from build123d import *

# Parameters (mm, degrees)
F0_R     = 25.4
F1_DEPTH = 12.7


with BuildPart() as f1:
    # F0 (on Front) → F1 (new body)
    with BuildSketch(Plane.XZ):
        with BuildLine():
            Line((31.8990597447, -65.5396825397), (36.8832878298, -2.9365079365))
            ThreePointArc((36.8832878298, -2.9365079365), (0, 37), (-36.8832878298, -2.9365079365))
            Line((-36.8832878298, -2.9365079365), (-31.8990597447, -65.5396825397))
            ThreePointArc((-31.8990597447, -65.5396825397), (0, -95), (31.8990597447, -65.5396825397))
        make_face()
        with BuildLine():
            Line((-17, -64.5), (-17, -61.5))
            ThreePointArc((-17, -61.5), (0, -44.5), (17, -61.5))
            Line((17, -61.5), (17, -64.5))
            ThreePointArc((17, -64.5), (0, -81.5), (-17, -64.5))
        make_face(mode=Mode.SUBTRACT)
        Circle(F0_R, mode=Mode.SUBTRACT)
    extrude(amount=F1_DEPTH)


solid = f1.part
Model file for the job. Use its own axes, mm. A direction names the side the tool comes from. Give positions to 0.01 mm unless a question says otherwise; leave off trailing zeros. Loops run counter-clockwise (first coordinate to the right, second up) from the corner with the lowest first, then second, coordinate; pieces in that order, holes last. Notation, with made-up numbers: (-12, 51.25) -> (25, 51.25) arc R12 ccw to (25, 66.25) -> close; hole circle Ø3 at (72, 46.5). An arc over 180 degrees is marked (long way). Use a Markdown table: item, result. Add a question column.
(1) Drop flat-ended pins along their axis: pin 1 Ø3 at (x, y) = (-5.5, -1.5) entering from +Z; pin 2 Ø2 at (y, z) = (-6, -24.5) entering from -X; pin 3 Ø2 at (x, y) = (9.5, -6.5) entering from +Z. Give the stop position or say it passes through.
(2) Slice it at B-B on z = -78. List the corners of the cut face in (x, y).
(3) Slice it at A-A on x = 0. List the corners of the cut face in (y, z).
(4) Mould opens along X. For faces 3 (the cylindrical face through (-5.506, -6.261, -24.796)), 4 (the flat face through (-1, 0, -28)), 5 (the cylindrical face through (0.374, -6.261, -81.496)), 6 (the cylindrical face through (0.85, -6.26, 36.99)) say: +X half, -X half, draft (parallel to the pull), parting line (faces both ways), or undercut.
(5) Slice it at C-C on y = -3. List the corners of the cut face in (x, z).
(6) Wall check: line 1 along Z through (x, y) = (-1, -11.5); line 2 along Z through (x, y) = (-9, -10); line 3 along Z through (x, y) = (19.5, -11). Give the ranges that are in metal, low to high.
(7) Slice it at D-D on x = 12. List the corners of the cut face in (y, z).
(8) Tool access for faces 1 (the flat face through (17, -6, -63)), 2 (the flat face through (-34.426, -6.261, -33.8)): list every direction of +Z, -Z, +X, -X, +Y, -Y with a clear straight run to the whole face (end or side of a thin tool).
Filled sheet:
| question | item | result |
|---|---|---|
| 1 | pin 1 | z = 36.78 |
| 1 | pin 2 | x = -35.25 |
| 1 | pin 3 | z = 36.01 |
| 2 | outline | (-28.27, -12.7) -> (-10.33, -12.7) -> (-10.33, 0) -> (-28.27, 0) -> close; (10.33, -12.7) -> (28.27, -12.7) -> (28.27, 0) -> (10.33, 0) -> close |
| 3 | outline | (-12.7, -95) -> (0, -95) -> (0, -81.5) -> (-12.7, -81.5) -> close; (-12.7, -44.5) -> (0, -44.5) -> (0, -25.4) -> (-12.7, -25.4) -> close; (-12.7, 25.4) -> (0, 25.4) -> (0, 37) -> (-12.7, 37) -> close |
| 4 | face 3 | undercut |
| 4 | face 4 | draft |
| 4 | face 5 | undercut |
| 4 | face 6 | parting line |
| 5 | outline | (-36.88, -2.94) -> (-31.9, -65.54) arc R32 ccw to (31.9, -65.54) -> (36.88, -2.94) arc R37 ccw (long way) to start; hole circle Ø50.8 at (0, 0); hole (-17, -64.5) arc R17 ccw to (17, -64.5) -> (17, -61.5) arc R17 ccw to (-17, -61.5) -> close |
| 6 | line 1 | -94.98 to -81.47, -44.53 to -25.38, 25.38 to 36.99 |
| 6 | line 2 | -93.71 to -78.92, -47.08 to -23.75, 23.75 to 35.89 |
| 6 | line 3 | -88.37 to -16.28, 16.28 to 31.44 |
| 7 | outline | (-12.7, -92.66) -> (0, -92.66) -> (0, -76.54) -> (-12.7, -76.54) -> close; (-12.7, -49.46) -> (0, -49.46) -> (0, -22.39) -> (-12.7, -22.39) -> close; (-12.7, 22.39) -> (0, 22.39) -> (0, 35) -> (-12.7, 35) -> close |
| 8 | face 1 | +Y, -Y |
| 8 | face 2 | -Z, -X, +Y, -Y |
